Autodesk Inventor part; units mm, degrees
ref_plane "YZ Plane" through (0, 0, 0) normal (1, 0, 0) x (0, 1, 0)
ref_plane "XZ Plane" through (0, 0, 0) normal (0, 1, 0) x (-1, 0, 0)
ref_plane "XY Plane" through (0, 0, 0) normal (0, 0, 1) x (1, 0, 0)
sketch "스케치1" plane through (0, 0, 0) normal (0, 1, 0) x (-1, 0, 0)
  line L0 (-32.5919, 13.5) -> (-13.5, 32.5919)
  line L1 (-13.5, 32.5919) -> (13.5, 32.5919)
  line L2 (13.5, 32.5919) -> (32.5919, 13.5)
  line L3 (32.5919, 13.5) -> (32.5919, -13.5)
  line L4 (32.5919, -13.5) -> (13.5, -32.5919)
  line L5 (13.5, -32.5919) -> (-13.5, -32.5919)
  line L6 (-13.5, -32.5919) -> (-32.5919, -13.5)
  line L7 (-32.5919, -13.5) -> (-32.5919, 13.5)
  line L8 (34.9919, 14.4941) -> (34.9919, -14.4941)
  line L9 (34.9919, -14.4941) -> (14.4941, -34.9919)
  line L10 (14.4941, -34.9919) -> (-14.4941, -34.9919)
  line L11 (-14.4941, -34.9919) -> (-34.9919, -14.4941)
  line L12 (-34.9919, -14.4941) -> (-34.9919, 14.4941)
  line L13 (-34.9919, 14.4941) -> (-14.4941, 34.9919)
  line L14 (-14.4941, 34.9919) -> (14.4941, 34.9919)
  line L15 (14.4941, 34.9919) -> (34.9919, 14.4941)
  point P0 (0, 0)
  point P1 (0, 0)
  point P2 (0, 0)
  dimension "d0" = 27
  dimension "d1" = 2.4
extrude "돌출1" add sketch "스케치1" along normal blind 3.4 contours L0 L1 L2 L3 L4 L5 L6 L7 | L8 L9 L10 L11 L12 L13 L14 L15
sketch "스케치2" plane through (0, 3.4, 0) normal (0, 1, 0) x (1, 0, 0)
  line L0 (13.5, -32.5919) -> (-13.5, -32.5919)
  line L1 (-13.5, -32.5919) -> (-32.5919, -13.5)
  line L2 (-32.5919, -13.5) -> (-32.5919, 13.5)
  line L3 (-32.5919, 13.5) -> (-13.5, 32.5919)
  line L4 (-13.5, 32.5919) -> (13.5, 32.5919)
  line L5 (13.5, 32.5919) -> (32.5919, 13.5)
  line L6 (32.5919, 13.5) -> (32.5919, -13.5)
  line L7 (32.5919, -13.5) -> (13.5, -32.5919)
  line L8 (-13.9971, -33.7919) -> (-33.7919, -13.9971)
  line L9 (-33.7919, -13.9971) -> (-33.7919, 13.9971)
  line L10 (-33.7919, 13.9971) -> (-13.9971, 33.7919)
  line L11 (-13.9971, 33.7919) -> (13.9971, 33.7919)
  line L12 (13.9971, 33.7919) -> (33.7919, 13.9971)
  line L13 (33.7919, 13.9971) -> (33.7919, -13.9971)
  line L14 (33.7919, -13.9971) -> (13.9971, -33.7919)
  line L15 (13.9971, -33.7919) -> (-13.9971, -33.7919)
  line L16 (-13.1686, 31.7919) -> (13.1686, 31.7919)
  line L17 (13.1686, 31.7919) -> (31.7919, 13.1686)
  line L18 (31.7919, 13.1686) -> (31.7919, -13.1686)
  line L19 (31.7919, -13.1686) -> (13.1686, -31.7919)
  line L20 (13.1686, -31.7919) -> (-13.1686, -31.7919)
  line L21 (-13.1686, -31.7919) -> (-31.7919, -13.1686)
  line L22 (-31.7919, -13.1686) -> (-31.7919, 13.1686)
  line L23 (-31.7919, 13.1686) -> (-13.1686, 31.7919)
  point P0 (0, 0)
  point P1 (0, 0)
  point P2 (0, 0)
  point P3 (0, 0)
  dimension "d4" = 27
  dimension "d5" = 1.2
  dimension "d16" = 0.8
sketch "스케치3" plane through (0, 0, 0) normal (0, -1, 0) x (1, 0, 0)
  line L0 (-13.5, 32.5919) -> (13.5, 32.5919)
  line L1 (13.5, 32.5919) -> (32.5919, 13.5)
  line L2 (32.5919, 13.5) -> (32.5919, -13.5)
  line L3 (32.5919, -13.5) -> (13.5, -32.5919)
  line L4 (13.5, -32.5919) -> (-13.5, -32.5919)
  line L5 (-13.5, -32.5919) -> (-32.5919, -13.5)
  line L6 (-32.5919, -13.5) -> (-32.5919, 13.5)
  line L7 (-32.5919, 13.5) -> (-13.5, 32.5919)
  line L8 (-13.9971, 33.7919) -> (13.9971, 33.7919)
  line L9 (13.9971, 33.7919) -> (33.7919, 13.9971)
  line L10 (33.7919, 13.9971) -> (33.7919, -13.9971)
  line L11 (33.7919, -13.9971) -> (13.9971, -33.7919)
  line L12 (13.9971, -33.7919) -> (-13.9971, -33.7919)
  line L13 (-13.9971, -33.7919) -> (-33.7919, -13.9971)
  line L14 (-33.7919, -13.9971) -> (-33.7919, 13.9971)
  line L15 (-33.7919, 13.9971) -> (-13.9971, 33.7919)
  line L16 (-13.1686, 31.7919) -> (13.1686, 31.7919)
  line L17 (13.1686, 31.7919) -> (31.7919, 13.1686)
  line L18 (31.7919, 13.1686) -> (31.7919, -13.1686)
  line L19 (31.7919, -13.1686) -> (13.1686, -31.7919)
  line L20 (13.1686, -31.7919) -> (-13.1686, -31.7919)
  line L21 (-13.1686, -31.7919) -> (-31.7919, -13.1686)
  line L22 (-31.7919, -13.1686) -> (-31.7919, 13.1686)
  line L23 (-31.7919, 13.1686) -> (-13.1686, 31.7919)
  point P0 (0, 0)
  point P1 (0, 0)
  point P2 (0, 0)
  point P3 (0, 0)
  dimension "d8" = 27
  dimension "d9" = 1.2
  dimension "d19" = 0.8
extrude "돌출3" cut sketch "스케치3" against normal blind 1.2 contours L0 L1 L2 L3 L4 L5 L6 L7 | L8 L9 L10 L11 L12 L13 L14 L15
sketch "스케치4" plane through (0, 3.4, 0) normal (0, 1, 0) x (1, 0, 0)
  line L0 (10.3934, -25.0919) -> (-10.3934, -25.0919)
  line L1 (-10.3934, -25.0919) -> (-25.0919, -10.3934)
  line L2 (-25.0919, -10.3934) -> (-25.0919, 10.3934)
  line L3 (-25.0919, 10.3934) -> (-10.3934, 25.0919)
  line L4 (-10.3934, 25.0919) -> (10.3934, 25.0919)
  line L5 (10.3934, 25.0919) -> (25.0919, 10.3934)
  line L6 (25.0919, 10.3934) -> (25.0919, -10.3934)
  line L7 (25.0919, -10.3934) -> (10.3934, -25.0919)
  point P0 (0, 0)
  point P1 (0, 0)
  dimension "d20" = 20.7868
extrude "돌출4" cut sketch "스케치4" against normal blind 5
extrude "돌출5" cut sketch "스케치2" against normal blind 1.2 contours L0 L1 L2 L3 L4 L5 L6 L7 | L8 L9 L10 L11 L12 L13 L14 L15
properties part number "팔각형 OV-PAM 5패턴 링 - 틈 너비 수정"
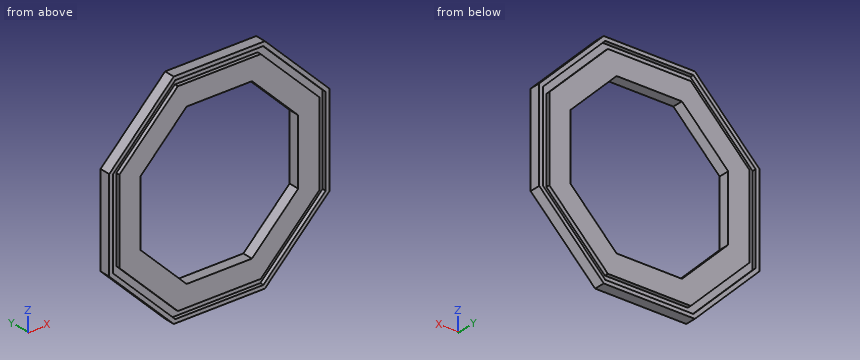
CAD build for the part. Positions are in the model's coordinates, mm. Coordinates: 2 decimals unless noted, no trailing zeros. Order: outer loops, then holes, each group sorted by start corner. A loop starts at its lowest first (then second) coordinate and runs counter-clockwise, first axis right, second up. Notation, with made-up numbers: (14, -10) -> (61, -10) arc R7 ccw to (61, 0) -> close; hole circle Ø6 at (19, 48). An arc over 180 degrees is marked (long way). Use one line per item in the form item = value. Start each with the question number.
1) Band-saw the part on C-C on z = -4.5. Give the cut face in (x, y), then the cut area to 3 significant figures.
2) Band-saw the part on A-A on y = 0.55. State how many separate pieces and enclosed holes the cut face has, then the cut area to 3 significant figures.
3) Band-saw the part on D-D on x = -29.5. Give the cut face in (y, z), then the cut area to 3 significant figures.
4) Drop a flat-ended pin along its axis: pin 1 (8 mm diameter, centred on x = -4, z = -17.5, fed in from +Y). Give the stop position or say it passes through.
5) Drill centre lines: L1, parallel to X at y = 0.55, z = 6.5; L2, parallel to X at y = 1.75, z = 2.5. Where is each one in solid material? Low to high. Write a range as [from, to].
6) Band-saw the part on B-B on x = 0. Give the cut face in (y, z).
Entries:
q1.outline = (-34.99, 0) -> (-33.79, 0) -> (-33.79, 1.2) -> (-31.79, 1.2) -> (-31.79, 0) -> (-25.09, 0) -> (-25.09, 3.4) -> (-31.79, 3.4) -> (-31.79, 2.2) -> (-33.79, 2.2) -> (-33.79, 3.4) -> (-34.99, 3.4) -> close; (25.09, 0) -> (31.79, 0) -> (31.79, 1.2) -> (33.79, 1.2) -> (33.79, 0) -> (34.99, 0) -> (34.99, 3.4) -> (33.79, 3.4) -> (33.79, 2.2) -> (31.79, 2.2) -> (31.79, 3.4) -> (25.09, 3.4) -> close
q1.area = 57.7 mm2
q2.separate_pieces = 2
q2.enclosed_holes = 2
q2.area = 1,540 mm2
q3.outline = (0, -19.99) -> (3.4, -19.99) -> (3.4, -18.29) -> (2.2, -18.29) -> (2.2, -15.46) -> (3.4, -15.46) -> (3.4, 15.46) -> (2.2, 15.46) -> (2.2, 18.29) -> (3.4, 18.29) -> (3.4, 19.99) -> (0, 19.99) -> (0, 18.29) -> (1.2, 18.29) -> (1.2, 15.46) -> (0, 15.46) -> (0, -15.46) -> (1.2, -15.46) -> (1.2, -18.29) -> (0, -18.29) -> close
q3.area = 122 mm2
q4.pin_1 = through
q5.L1 = [-34.99, -33.79], [-31.79, -25.09], [25.09, 31.79], [33.79, 34.99]
q5.L2 = [-34.99, -25.09], [25.09, 34.99]
q6.outline = (0, -34.99) -> (3.4, -34.99) -> (3.4, -33.79) -> (2.2, -33.79) -> (2.2, -31.79) -> (3.4, -31.79) -> (3.4, -25.09) -> (0, -25.09) -> (0, -31.79) -> (1.2, -31.79) -> (1.2, -33.79) -> (0, -33.79) -> close; (0, 25.09) -> (3.4, 25.09) -> (3.4, 31.79) -> (2.2, 31.79) -> (2.2, 33.79) -> (3.4, 33.79) -> (3.4, 34.99) -> (0, 34.99) -> (0, 33.79) -> (1.2, 33.79) -> (1.2, 31.79) -> (0, 31.79) -> close
